Verification items for the finished model (mm, model axes). Round coordinates to 2 decimals unless told otherwise and drop trailing zeros. Order: outer loops, then holes, each group sorted by start corner. A loop starts at its lowest first (then second) coordinate and runs counter-clockwise, first axis right, second up. Notation, with made-up numbers: (60.5, 86) -> (102.5, 86) arc R18 cw to (102.5, 118) -> close; hole circle Ø3 at (44.25, -20.5). An arc over 180 degrees is marked (long way). Write item = value, one per line. Start each with the question number.
from build123d import *

# Parameters (mm, degrees)
F0_R     = 12.5
F1_DEPTH = 148


with BuildPart() as f1:
    # F0 (on Top) → F1 (new body)
    with BuildSketch(Plane.XY):
        Circle(F0_R)
        with BuildLine():
            ThreePointArc((5.5303976568, 2.3269511721), (5.8814278003, 1.1869317712), (6, 0))
            ThreePointArc((6, 0), (5.8814278003, -1.1869317712), (5.5303976568, -2.3269511721))
            Line((5.5303976568, -2.3269511721), (5.5711524227, -2.3504809472))
            Line((5.5711524227, -2.3504809472), (5.1961523876, -3.0000000609))
            Line((5.1961523876, -3.0000000609), (4.8211524227, -3.6495190528))
            Line((4.8211524227, -3.6495190528), (4.7803976568, -3.6259892778))
            ThreePointArc((4.7803976568, -3.6259892778), (3, -5.1961524227), (0.75, -5.9529404499))
            Line((0.75, -5.9529404499), (0.75, -6))
            Line((0.75, -6), (0, -6))
            Line((0, -6), (-0.75, -6))
            Line((-0.75, -6), (-0.75, -5.9529404499))
            ThreePointArc((-0.75, -5.9529404499), (-3, -5.1961524227), (-4.7803976568, -3.6259892778))
            Line((-4.7803976568, -3.6259892778), (-4.8211524227, -3.6495190528))
            Line((-4.8211524227, -3.6495190528), (-5.1961524003, -3.0000000387))
            Line((-5.1961524003, -3.0000000387), (-5.5711524227, -2.3504809472))
            Line((-5.5711524227, -2.3504809472), (-5.5303976568, -2.3269511721))
            ThreePointArc((-5.5303976568, -2.3269511721), (-6, 0), (-5.5303976568, 2.3269511721))
            Line((-5.5303976568, 2.3269511721), (-5.5711524227, 2.3504809472))
            Line((-5.5711524227, 2.3504809472), (-5.1961524003, 3.0000000387))
            Line((-5.1961524003, 3.0000000387), (-4.8211524227, 3.6495190528))
            Line((-4.8211524227, 3.6495190528), (-4.7803976568, 3.6259892778))
            ThreePointArc((-4.7803976568, 3.6259892778), (-3, 5.1961524227), (-0.75, 5.9529404499))
            Line((-0.75, 5.9529404499), (-0.75, 6))
            Line((-0.75, 6), (0, 6))
            Line((0, 6), (0.75, 6))
            Line((0.75, 6), (0.75, 5.9529404499))
            ThreePointArc((0.75, 5.9529404499), (3, 5.1961524227), (4.7803976568, 3.6259892778))
            Line((4.7803976568, 3.6259892778), (4.8211524227, 3.6495190528))
            Line((4.8211524227, 3.6495190528), (5.1961524003, 3.0000000387))
            Line((5.1961524003, 3.0000000387), (5.5711524227, 2.3504809472))
            Line((5.5711524227, 2.3504809472), (5.5303976568, 2.3269511721))
        make_face(mode=Mode.SUBTRACT)
        with BuildLine():
            Line((-3.0891016151, 2.6495190528), (-4.7803976568, 3.6259892778))
            ThreePointArc((-4.7803976568, 3.6259892778), (-4.9980849725, 3.3195099951), (-5.1961524003, 3.0000000387))
            ThreePointArc((-5.1961524003, 3.0000000387), (-5.3738224502, 2.668713599), (-5.5303976568, 2.3269511721))
            Line((-5.5303976568, 2.3269511721), (-3.8391016151, 1.3504809472))
            Line((-3.8391016151, 1.3504809472), (-3.0891016151, 2.6495190528))
        make_face()
        with BuildLine():
            Line((0.75, 4), (0.75, 5.9529404499))
            ThreePointArc((0.75, 5.9529404499), (0.3757374753, 5.9882235554), (0, 6))
            ThreePointArc((0, 6), (-0.3757374753, 5.9882235554), (-0.75, 5.9529404499))
            Line((-0.75, 5.9529404499), (-0.75, 4))
            Line((-0.75, 4), (0.75, 4))
        make_face()
        with BuildLine():
            Line((3.8391016151, 1.3504809472), (5.5303976568, 2.3269511721))
            ThreePointArc((5.5303976568, 2.3269511721), (5.3738224502, 2.668713599), (5.1961524003, 3.0000000387))
            ThreePointArc((5.1961524003, 3.0000000387), (4.9980849725, 3.3195099951), (4.7803976568, 3.6259892778))
            Line((4.7803976568, 3.6259892778), (3.0891016151, 2.6495190528))
            Line((3.0891016151, 2.6495190528), (3.8391016151, 1.3504809472))
        make_face()
        with BuildLine():
            ThreePointArc((5.1961523876, -3.0000000609), (5.3738224445, -2.6687136105), (5.5303976568, -2.3269511721))
            Line((5.5303976568, -2.3269511721), (3.8391016151, -1.3504809472))
            Line((3.8391016151, -1.3504809472), (3.0891016151, -2.6495190528))
            Line((3.0891016151, -2.6495190528), (4.7803976568, -3.6259892778))
            ThreePointArc((4.7803976568, -3.6259892778), (4.9980849655, -3.3195100057), (5.1961523876, -3.0000000609))
        make_face()
        with BuildLine():
            ThreePointArc((0, -6), (0.3757374753, -5.9882235554), (0.75, -5.9529404499))
            Line((0.75, -5.9529404499), (0.75, -4))
            Line((0.75, -4), (-0.75, -4))
            Line((-0.75, -4), (-0.75, -5.9529404499))
            ThreePointArc((-0.75, -5.9529404499), (-0.3757374753, -5.9882235554), (0, -6))
        make_face()
        with BuildLine():
            ThreePointArc((-5.1961524003, -3.0000000387), (-4.9980849725, -3.3195099951), (-4.7803976568, -3.6259892778))
            Line((-4.7803976568, -3.6259892778), (-3.0891016151, -2.6495190528))
            Line((-3.0891016151, -2.6495190528), (-3.8391016151, -1.3504809472))
            Line((-3.8391016151, -1.3504809472), (-5.5303976568, -2.3269511721))
            ThreePointArc((-5.5303976568, -2.3269511721), (-5.3738224502, -2.668713599), (-5.1961524003, -3.0000000387))
        make_face()
        with BuildLine():
            ThreePointArc((0, 6), (0.3757374753, 5.9882235554), (0.75, 5.9529404499))
            Line((0.75, 5.9529404499), (0.75, 6))
            Line((0.75, 6), (0, 6))
        make_face()
        with BuildLine():
            ThreePointArc((-0.75, 5.9529404499), (-0.3757374753, 5.9882235554), (0, 6))
            Line((0, 6), (-0.75, 6))
            Line((-0.75, 6), (-0.75, 5.9529404499))
        make_face()
        with BuildLine():
            ThreePointArc((-5.1961524003, 3.0000000387), (-4.9980849725, 3.3195099951), (-4.7803976568, 3.6259892778))
            Line((-4.7803976568, 3.6259892778), (-4.8211524227, 3.6495190528))
            Line((-4.8211524227, 3.6495190528), (-5.1961524003, 3.0000000387))
        make_face()
        with BuildLine():
            ThreePointArc((4.7803976568, 3.6259892778), (4.9980849725, 3.3195099951), (5.1961524003, 3.0000000387))
            Line((5.1961524003, 3.0000000387), (4.8211524227, 3.6495190528))
            Line((4.8211524227, 3.6495190528), (4.7803976568, 3.6259892778))
        make_face()
        with BuildLine():
            Line((0.75, -6), (0.75, -5.9529404499))
            ThreePointArc((0.75, -5.9529404499), (0.3757374753, -5.9882235554), (0, -6))
            Line((0, -6), (0.75, -6))
        make_face()
        with BuildLine():
            Line((4.8211524227, -3.6495190528), (5.1961523876, -3.0000000609))
            ThreePointArc((5.1961523876, -3.0000000609), (4.9980849655, -3.3195100057), (4.7803976568, -3.6259892778))
            Line((4.7803976568, -3.6259892778), (4.8211524227, -3.6495190528))
        make_face()
        with BuildLine():
            ThreePointArc((5.1961524003, 3.0000000387), (5.3738224502, 2.668713599), (5.5303976568, 2.3269511721))
            Line((5.5303976568, 2.3269511721), (5.5711524227, 2.3504809472))
            Line((5.5711524227, 2.3504809472), (5.1961524003, 3.0000000387))
        make_face()
        with BuildLine():
            ThreePointArc((-5.5303976568, 2.3269511721), (-5.3738224502, 2.668713599), (-5.1961524003, 3.0000000387))
            Line((-5.1961524003, 3.0000000387), (-5.5711524227, 2.3504809472))
            Line((-5.5711524227, 2.3504809472), (-5.5303976568, 2.3269511721))
        make_face()
        with BuildLine():
            Line((-5.5711524227, -2.3504809472), (-5.1961524003, -3.0000000387))
            ThreePointArc((-5.1961524003, -3.0000000387), (-5.3738224502, -2.668713599), (-5.5303976568, -2.3269511721))
            Line((-5.5303976568, -2.3269511721), (-5.5711524227, -2.3504809472))
        make_face()
        with BuildLine():
            Line((-4.8211524227, -3.6495190528), (-4.7803976568, -3.6259892778))
            ThreePointArc((-4.7803976568, -3.6259892778), (-4.9980849725, -3.3195099951), (-5.1961524003, -3.0000000387))
            Line((-5.1961524003, -3.0000000387), (-4.8211524227, -3.6495190528))
        make_face()
        with BuildLine():
            Line((-0.75, -6), (0, -6))
            ThreePointArc((0, -6), (-0.3757374753, -5.9882235554), (-0.75, -5.9529404499))
            Line((-0.75, -5.9529404499), (-0.75, -6))
        make_face()
        with BuildLine():
            Line((5.5711524227, -2.3504809472), (5.5303976568, -2.3269511721))
            ThreePointArc((5.5303976568, -2.3269511721), (5.3738224445, -2.6687136105), (5.1961523876, -3.0000000609))
            Line((5.1961523876, -3.0000000609), (5.5711524227, -2.3504809472))
        make_face()
    extrude(amount=F1_DEPTH)


solid = f1.part
(1) Depth check by flat-ended pin: pin 1 (1.6 mm diameter, centred on y = 5, z = 83, fed in from +X); pin 2 (8 mm diameter, centred on x = 9.5, z = 17, fed in from -Y) (3 decimals); pin 3 (2 mm diameter, centred on y = 5, z = 53.5, fed in from -X). Enter the tip coordinate at first touch or a pass-through.
(2) Scan lines: line 1 along X through (y, z) = (-0.25, 83); line 2 along Y through (x, z) = (3.25, 89); line 3 along Y through (x, z) = (0.5, 43.5). Record each from-to range of solid material in increasing order. Write a range as from..to.
(3) Cross-section at B-B (x = 9.75). Enter the section's corners in (y, z).
(4) Draft check along X on faces 1 (the flat face through (0, -5, 0)), 2 (the cylindrical face through (11.923, 3.755, 72.964)), 3 (the cylindrical face through (-6, 0, 73)). Enter one of: +X half, -X half, draft (parallel to the pull), parting line (faces both ways), or undercut.
(5) Cross-section at C-C (x = -8). Enter the section's corners in (y, z).
(6) Cross-section at A-A (z = 65). Enter the section's corners in (x, y), and give its area (3 significant figures).
Outcome:
q1.pin_1 = 11.77
q1.pin_2 = -11.225
q1.pin_3 = -11.84
q2.line_1 = -12.5..-5.99, 5.99..12.5
q2.line_2 = -12.07..-5.04, -2.74..-2.37, 2.37..2.74, 5.04..12.07
q2.line_3 = -12.49..-4, 4..12.49
q3.outline = (-7.82, 0) -> (7.82, 0) -> (7.82, 148) -> (-7.82, 148) -> close
q4.face_1 = draft
q4.face_2 = parting line
q4.face_3 = undercut
q5.outline = (-9.6, 0) -> (9.6, 0) -> (9.6, 148) -> (-9.6, 148) -> close
q6.outline = circle Ø25 at (0, 0); hole (-5.53, -2.33) -> (-3.84, -1.35) -> (-3.09, -2.65) -> (-4.78, -3.63) arc R6 ccw to (-0.75, -5.95) -> (-0.75, -4) -> (0.75, -4) -> (0.75, -5.95) arc R6 ccw to (4.78, -3.63) -> (3.09, -2.65) -> (3.84, -1.35) -> (5.53, -2.33) arc R6 ccw to (5.53, 2.33) -> (3.84, 1.35) -> (3.09, 2.65) -> (4.78, 3.63) arc R6 ccw to (0.75, 5.95) -> (0.75, 4) -> (-0.75, 4) -> (-0.75, 5.95) arc R6 ccw to (-4.78, 3.63) -> (-3.09, 2.65) -> (-3.84, 1.35) -> (-5.53, 2.33) arc R6 ccw to start
q6.area = 396 mm^2
